from build123d import *

# Parameters (mm, degrees)
F0_R     = 22.225
F0_R_2   = 19.05
F1_DEPTH = 76.2
F2_START = 73.025
F2_DEPTH = 3.175
F3_R     = 22.225
F3_R_2   = 19.05
F4_DEPTH = 35.9833333333
F5_DEPTH = 63.5
F6_DEPTH = 25.4
F7_DEPTH = 25.4
F8_DEPTH = 25.4


with BuildPart() as f1:
    # F0 (on Top) → F1 (new body)
    with BuildSketch(Plane.XY):
        Circle(F0_R)
        Circle(F0_R_2, mode=Mode.SUBTRACT)
    extrude(amount=F1_DEPTH)

    # F0 (on Top) → F2 (join)
    with BuildSketch(Plane.XY.offset(F2_START)):
        Circle(F0_R)
        Circle(F0_R_2, mode=Mode.SUBTRACT)
        Circle(F0_R_2)
    extrude(amount=F2_DEPTH)

    # F3 (on Right) → F4 (join)
    with BuildSketch(Plane.YZ):
        with Locations((0, 35.9833333333)):
            Circle(F3_R)
        with Locations((0, 35.9833333333)):
            Circle(F3_R_2, mode=Mode.SUBTRACT)
    extrude(amount=F4_DEPTH)

    # F0 (on Top) → F5 (cut)
    with BuildSketch(Plane.XY):
        Circle(F0_R_2)
    extrude(amount=F5_DEPTH, mode=Mode.SUBTRACT)

    # F3 (on Right) → F6 (cut)
    with BuildSketch(Plane.YZ):
        with Locations((0, 35.9833333333)):
            Circle(F3_R_2)
    extrude(amount=F6_DEPTH, mode=Mode.SUBTRACT)

    # F7 (add): a face of the model
    f7_faces = [f1.faces().sort_by_distance(p)[0] for p in [
        (35.9833333333, -21.5963820715, 35.9833333333),
    ]]
    extrude(f7_faces, amount=F7_DEPTH)

    # F8 (add): a face of the model
    f8_faces = [f1.faces().sort_by_distance(p)[0] for p in [
        (-21.5963820715, 0, 0),
    ]]
    extrude(f8_faces, amount=F8_DEPTH)


solid = f1.part
The model under review builds one solid part; all positions refer to its coordinate system, in mm. A direction names the side the tool comes from. Round coordinates to 2 decimals unless told otherwise and drop trailing zeros. Order: outer loops, then holes, each group sorted by start corner. A loop starts at its lowest first (then second) coordinate and runs counter-clockwise, first axis right, second up. Notation, with made-up numbers: (-27.5, 71) -> (18.5, 71) arc R12 cw to (18.5, 75) -> close; hole circle Ø9 at (-6, -18.5). An arc over 180 degrees is marked (long way). Use CSV: the item, a comma, the result in double quotes. Start each with the question number.
(1) Insertion check: pin 1 (3 mm diameter, centred on y = -7, z = -13.5, fed in from +X); pin 2 (11.5 mm diameter, centred on x = 5, y = 6.5, fed in from -Z) (3 decimals); pin 3 (10 mm diameter, centred on y = 16.5, z = 0, fed in from -X). Each pin has a flat end and moves straight along its axis. Give the tip position at first contact, or say it passes through.
(2) Consider section B-B on z = 40.5. Write out the cut boundary in (x, y) (3 decimals), and give its area (3 significant figures).
(3) Mouldability with a two-part tool opening along Y and no side actions: class faces 1 (the face through (37.1, -22.2, 37)), 2 (the face through (-19.03, 0.84, 23.12)), 3 (the face through (61.383, 16.4, 46)) as pulls with the +Y half, pulls with the -Y half, needs draft (parallel to the pull), parting line crosses it, or undercut.
(4) Consider section C-C on x = -3.5. Write out the cut boundary in (y, z) (3 decimals).
(5) Wall thickness on probe 1 along Z at (x, y) = (29, 0); probe 2 along Z at (x, y) = (19.5, 1); probe 3 along Y at (x, z) = (52, 37): over which ranges is each line inside the solid? List them lowest first. Write a range as from..to.
(6) Consider section A-A on y = 0. Write out the cut boundary in (x, z) (3 decimals).
(7) Consider section D-D on z = 9. Write out the cut boundary in (x, y) (3 decimals), and give its area (3 significant figures).
(8) Tool access review of faces 4 (the face through (37.08, -2.48, 54.87)), 5 (the face through (0, 0, 73.025)), 6 (the face through (-22.204, 0.977, 26.111)): name each direction out of +Z, -Z, +X, -X, +Y, -Y from which nothing blocks a thin tool from reaching the whole face with its end or side.
Responses:
1,pin 1,"x = 21.53"
1,pin 2,"z = 73.025"
1,pin 3,"x = -19.02"
2,outline,"(4.517, -21.761) -> (61.383, -21.761) -> (61.383, -18.507) -> (4.517, -18.507) arc R19.05 cw (long way) to (4.517, 18.507) -> (61.383, 18.507) -> (61.383, 21.761) -> (4.517, 21.761) arc R22.225 ccw (long way) to start"
2,area,"605 mm²"
3,face 1,"parting line crosses it"
3,face 2,"undercut"
3,face 3,"needs draft"
4,outline,"(-21.948, -25.4) -> (-18.726, -25.4) -> (-18.726, 73.025) -> (18.726, 73.025) -> (18.726, -25.4) -> (21.948, -25.4) -> (21.948, 76.2) -> (-21.948, 76.2) -> close"
5,probe 1,"13.76..16.93, 55.03..58.21"
5,probe 2,"-25.4..16.96, 55.01..76.2"
5,probe 3,"-22.2..-19.02, 19.02..22.2"
6,outline,"(-22.225, -25.4) -> (-19.05, -25.4) -> (-19.05, 73.025) -> (19.05, 73.025) -> (19.05, 55.033) -> (61.383, 55.033) -> (61.383, 58.208) -> (22.225, 58.208) -> (22.225, 76.2) -> (-22.225, 76.2) -> close; (19.05, -25.4) -> (22.225, -25.4) -> (22.225, 13.758) -> (61.383, 13.758) -> (61.383, 16.933) -> (19.05, 16.933) -> close"
7,outline,"circle Ø44.45 at (0, 0); hole circle Ø38.1 at (0, 0)"
7,area,"412 mm²"
8,face 4,"+X"
8,face 5,"-Z"
8,face 6,"none"
